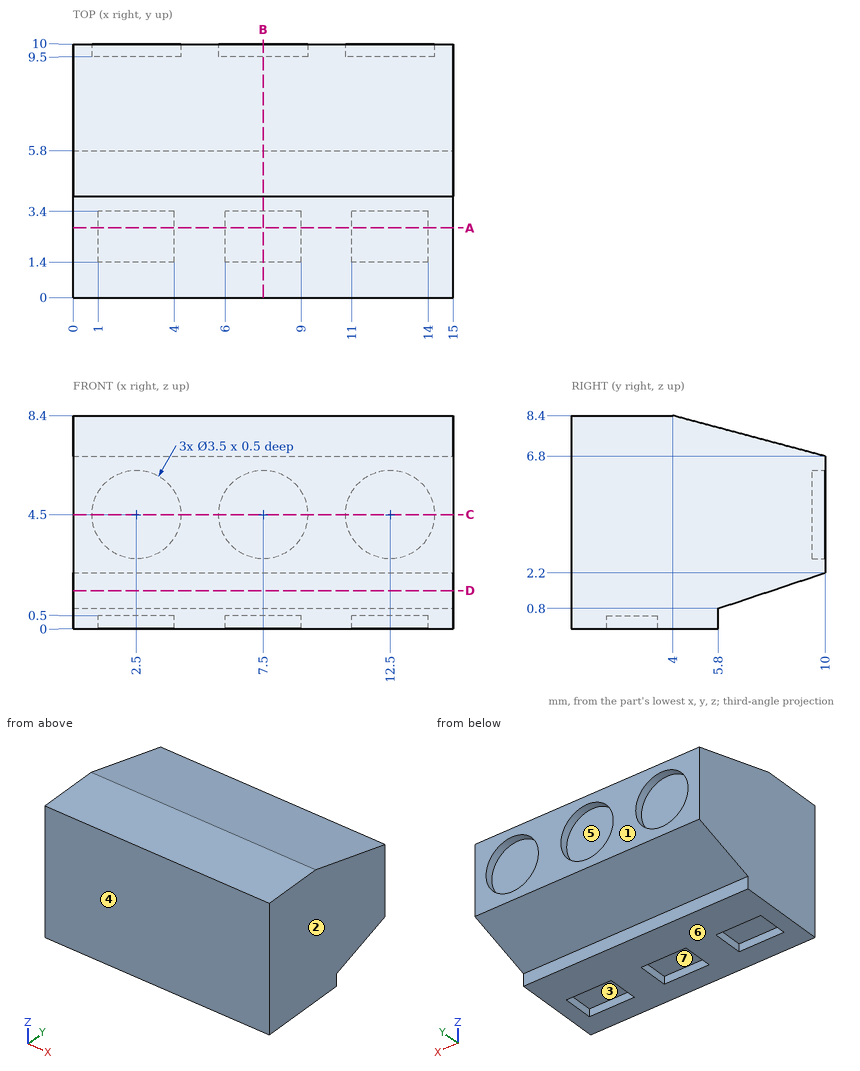
Job drawing, mm, ordinate dimensions from the low corner. One solid piece. A direction names the side the tool comes from. Round coordinates to 2 decimals unless told otherwise and drop trailing zeros. Write each loop counter-clockwise with the first axis right and the second up, starting at its lowest first coordinate (ties: lowest second). Pieces come first, ordered by that corner, then holes. Notation, with made-up numbers: M 40,67.25 L 65,67.25 A16 ccw 65,81.25 Z; hole C -33,38 d11. An arc over 180 degrees is marked long. Return JSON: item names as keys, results as strings. Group by question number.
(1) Two-plate mould, pull along Y, no slides. Class the marked faces 1, 2, 3 and 4: +Y half, -Y half, draft (parallel to the pull), parting line (faces both ways), or undercut.
(2) Drill centre lines: probe 1 along X at (y, z) = (9.65, 4.5); probe 2 along Y at (x, z) = (8.25, 6); probe 3 along Z at (x, y) = (7.5, 9.8). Where is each one in solid material? Low to high.
(3) Saw through at A-A on y = 2.75. Write the cut outline in (x, z).
(4) Which spindle directions (+Z, -Z, +X, -X, +Y, -Y) get a long thin tool onto all of the face, cutting with end or side? Do the marked faces 5, 6 and 7. Say none if no direction does.
(5) Pin check, flat tips, straight feed: pin 1 Ø1 at (x, y) = (13, 2.5) entering from -Z; pin 2 Ø4 at (x, z) = (8, 3.5) entering from +Y; pin 3 Ø1 at (x, z) = (8, 4) entering from +Y; pin 4 Ø1 at (x, y) = (6, 6.5) entering from -Z. Stop position of each tip, or through.
(6) Saw through at C-C on z = 4.5. Write the cut outline in (x, y).
(7) Saw through at D-D on z = 1.5. Write the cut outline in (x, y), then the cut area to 4 significant figures.
(8) Saw through at B-B on x = 7.5. Write the cut outline in (y, z), then the cut area to 4 significant figures.
Returned:
{
 "1": {"face 1": "+Y half", "face 2": "draft", "face 3": "undercut", "face 4": "-Y half"},
 "2": {"probe 1": "0 to 0.75, 4.25 to 5.75, 9.25 to 10.75, 14.25 to 15", "probe 2": "0 to 9.5", "probe 3": "2.13 to 2.75, 6.25 to 6.85"},
 "3": {"outline": "M 0,0 L 1,0 L 1,0.5 L 4,0.5 L 4,0 L 6,0 L 6,0.5 L 9,0.5 L 9,0 L 11,0 L 11,0.5 L 14,0.5 L 14,0 L 15,0 L 15,8.4 L 0,8.4 Z"},
 "4": {"face 5": "+Y", "face 6": "-Z, +X, -X, +Y, -Y", "face 7": "-Z"},
 "5": {"pin 1": "z = 0.5", "pin 2": "y = 10", "pin 3": "y = 9.5", "pin 4": "z = 0.87"},
 "6": {"outline": "M 0,0 L 15,0 L 15,10 L 14.25,10 L 14.25,9.5 L 10.75,9.5 L 10.75,10 L 9.25,10 L 9.25,9.5 L 5.75,9.5 L 5.75,10 L 4.25,10 L 4.25,9.5 L 0.75,9.5 L 0.75,10 L 0,10 Z"},
 "7": {"outline": "M 0,0 L 15,0 L 15,7.9 L 0,7.9 Z", "area": "118.5 mm²"},
 "8": {"outline": "M 0,0 L 1.4,0 L 1.4,0.5 L 3.4,0.5 L 3.4,0 L 5.8,0 L 5.8,0.8 L 10,2.2 L 10,2.75 L 9.5,2.75 L 9.5,6.25 L 10,6.25 L 10,6.8 L 4,8.4 L 0,8.4 Z", "area": "70.15 mm²"}
}
